Here's how the part is built. I have some questions about the finished solid (model axes, mm). A direction names the side the tool comes from. Give positions to 0.01 mm unless a question says otherwise; leave off trailing zeros. Loops run counter-clockwise (first coordinate to the right, second up) from the corner with the lowest first, then second, coordinate; pieces in that order, holes last. Notation, with made-up numbers: (36, 34.25) -> (48, 34.25) arc R31 ccw to (48, 58.25) -> close; hole circle Ø3 at (75, 34.25). An arc over 180 degrees is marked (long way). Answer in a Markdown table with one row per item. Add a question column.
Item 1: If we section it at B-B (z = -0.9): Write out the boundary of the cut face in (x, y) (3 decimals), then the cut area to 3 significant figures.
Item 2: We'd pull the mould along Y, two halves only. Please class faces 1 (the face through (4.43, 2.43, -0.27)), 2 (the face through (7, -8, 0.33)): released by +Y, released by -Y, zero draft, split by the parting line, or undercut.
Item 3: If we section it at C-C (y = 8): Write out the boundary of the cut face in (x, z).
Item 4: For P1, Ø5, axis at x = -8, y = -6, coming from the +Z side, with a flat end and sliding along its axis, tell me the tip position at first contact or that it passes through.
Item 5: If we section it at A-A (x = 8.5): Write out the boundary of the cut face in (y, z).
Item 6: If we section it at D-D (x = 2.75): Write out the boundary of the cut face in (y, z), then the cut area to 3 significant figures.
Item 7: If I drill on line 1 (Y direction, x = 0, z = 0.1) (3 decimals); line 2 (Z direction, x = 5.75, y = 4.5); line 3 (Z direction, x = -5.25, y = -6), over which ranges is the centre line in solid material (lowest first)?
Item 8: Which directions (+Z, -Z, +X, -X, +Y, -Y) give clear straight access to the entire face, cutting with the end or side of a thin tool? Please do faces 3 (the face through (0, 0, -2)), 4 (the face through (0, 0, -0.27)).
```python
from build123d import *

# Parameters (mm, degrees)
SKETCH_R           = 11.625
PAD_DEPTH          = 2.33
SKETCH001_R        = 10.284193
POCKET_DEPTH       = 0.6
PAD001_DEPTH       = 0.3
POLARPATTERN_COUNT = 8


with BuildPart() as part:
    # Sketch → Pad (new body)
    with BuildSketch(Plane.XY):
        Circle(SKETCH_R)
    extrude(amount=PAD_DEPTH)

    # Sketch001 (on Face3 of Pad) → Pocket (cut)
    with BuildSketch(Plane.XY.offset(2.33)):
        Circle(SKETCH001_R)
    extrude(amount=-POCKET_DEPTH, mode=Mode.SUBTRACT)

    # Sketch002 (on Face5 of Pocket) → Pad001 (join)
    with BuildSketch(Plane.XY.offset(1.73)):
        with BuildLine():
            Line((-0.2, 4.495553), (-0.2, 6.326262))
            Line((-0.2, 6.326262), (-0.989949, 7.116211))
            ThreePointArc((-0.707107, 7.399054), (-0.989949, 7.399054), (-0.989949, 7.116211))
            Line((-0.707107, 7.399054), (0, 6.691947))
            Line((0, 6.691947), (0.707107, 7.399054))
            ThreePointArc((0.989949, 7.116211), (0.989949, 7.399054), (0.707107, 7.399054))
            Line((0.989949, 7.116211), (0.2, 6.326262))
            Line((0.2, 6.326262), (0.2, 4.895917))
            ThreePointArc((1.68881, 4.599774), (0.955943, 4.805848), (0.2, 4.895917))
            Line((1.68881, 4.599774), (1.909463, 5.132477))
            Line((1.909463, 5.132477), (1.481946, 6.164596))
            ThreePointArc((1.851498, 6.31767), (1.590185, 6.425909), (1.481946, 6.164596))
            Line((1.851498, 6.31767), (2.234181, 5.39379))
            Line((2.234181, 5.39379), (3.158061, 5.776474))
            ThreePointArc((3.311134, 5.406922), (3.419373, 5.668234), (3.158061, 5.776474))
            Line((3.311134, 5.406922), (2.279015, 4.979404))
            Line((2.279015, 4.979404), (2.058362, 4.446701))
            ThreePointArc((4.352946, 2.249858), (3.38862, 3.539386), (2.058362, 4.446701))
            Line((4.352946, 2.249858), (3.997604, 2.066196))
            ThreePointArc((3.997604, 2.066196), (2.254083, 3.894754), (-0.2, 4.495553))
        make_face()
    pad001 = extrude(amount=PAD001_DEPTH)

    # PolarPattern: Pad001 ×8 about axis
    polarpattern_axis = Axis((0, 0, 1.73), (0, 0, 1))
    for i in range(1, POLARPATTERN_COUNT):
        add(pad001.rotate(polarpattern_axis, i * 360 / POLARPATTERN_COUNT))


with BuildPart() as part_1:
    # Body placement: moved
    add(part.part.moved(Location((0, 0, -2))))


solid = part_1.part
```
Recorded:
| question | item | result |
|---|---|---|
| 1 | outline | circle Ø23.25 at (0, 0) |
| 1 | area | 425 mm^2 |
| 2 | face 1 | undercut |
| 2 | face 2 | zero draft |
| 3 | outline | (-8.43, -2) -> (8.43, -2) -> (8.43, 0.33) -> (6.46, 0.33) -> (6.46, -0.27) -> (-6.46, -0.27) -> (-6.46, 0.33) -> (-8.43, 0.33) -> close |
| 4 | P1 | stops at z = 0.33 |
| 5 | outline | (-7.93, -2) -> (7.93, -2) -> (7.93, 0.33) -> (5.79, 0.33) -> (5.79, -0.27) -> (-5.79, -0.27) -> (-5.79, 0.33) -> (-7.93, 0.33) -> close |
| 6 | outline | (-11.3, -2) -> (11.3, -2) -> (11.3, 0.33) -> (9.91, 0.33) -> (9.91, -0.27) -> (5.61, -0.27) -> (5.61, 0.03) -> (5.17, 0.03) -> (5.17, -0.27) -> (4.06, -0.27) -> (4.06, 0.03) -> (3.56, 0.03) -> (3.56, -0.27) -> (-3.56, -0.27) -> (-3.56, 0.03) -> (-4.06, 0.03) -> (-4.06, -0.27) -> (-5.17, -0.27) -> (-5.17, 0.03) -> (-5.61, 0.03) -> (-5.61, -0.27) -> (-9.91, -0.27) -> (-9.91, 0.33) -> (-11.3, 0.33) -> close |
| 6 | area | 41.3 mm^2 |
| 7 | line 1 | y = -11.625 to -10.284, 10.284 to 11.625 |
| 7 | line 2 | z = -2 to 0.03 |
| 7 | line 3 | z = -2 to -0.27 |
| 8 | face 3 | -Z, +X, -X, +Y, -Y |
| 8 | face 4 | +Z |
